CAD build for the part. Positions are in the model's coordinates, mm. Face numbers are marked on the shaded views. A direction names the side the tool comes from. Round coordinates to 2 decimals unless told otherwise and drop trailing zeros. Loops run counter-clockwise (first coordinate to the right, second up) from the corner with the lowest first, then second, coordinate; pieces in that order, holes last.
from build123d import *

# Parameters (mm, degrees)
SKETCH3_W           = 38.1
SKETCH3_H           = 41.932660102
SKETCH3_R           = 7.1501
BOSS_EXTRUDE1_DEPTH = 2.54
SKETCH4_W           = 8.89
SKETCH4_H           = 2.54
BOSS_EXTRUDE2_DEPTH = 8.89


with BuildPart() as part:
    # Sketch3 → Boss-Extrude1 (new body)
    with BuildSketch(Plane(origin=(-73.0954, 0, 0), x_dir=(0, 0, -1), z_dir=(1, 0, 0))):
        with Locations((0, -1.916330051)):
            Rectangle(SKETCH3_W, SKETCH3_H)
        Circle(SKETCH3_R, mode=Mode.SUBTRACT)
    extrude(amount=-BOSS_EXTRUDE1_DEPTH)

    # Sketch4 → Boss-Extrude2 (add)
    with BuildSketch(Plane(origin=(-73.0954, 0, 0), x_dir=(0, 0, -1), z_dir=(1, 0, 0))):
        with Locations((14.605, -21.612660102)):
            Rectangle(SKETCH4_W, SKETCH4_H)
        with Locations((-14.605, -21.612660102)):
            Rectangle(SKETCH4_W, SKETCH4_H)
    extrude(amount=-BOSS_EXTRUDE2_DEPTH)


solid = part.part
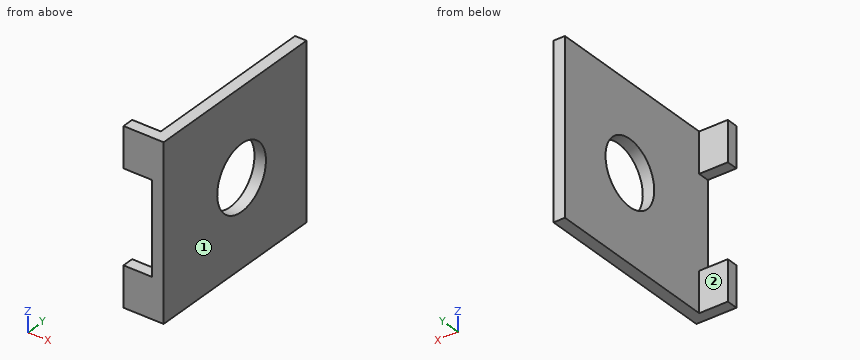
Item 1: Cut at D-D (y = 15.5). List the corners of the cut face in (x, z), plus the area to 3 significant figures.
Verdict:
outline: (-75.64, -19.05) - (-73.1, -19.05) - (-73.1, 19.05) - (-75.64, 19.05) - close
area: 96.8 mm2
Item 2: Wall check: L1, parallel to Y at x = -73.65, z = 0; L2, parallel to X at y = -4, z = 11; L3, parallel to Y at x = -75, z = -6. Give the ranges that are in metal, low to high.
Verdict:
L1: y = -22.88 to -7.15, 7.15 to 19.05
L2: x = -75.64 to -73.1
L3: y = -22.88 to -3.89, 3.89 to 19.05
Item 3: Flat gauge pins, fed straight in: P1, Ø1.9, axis at x = -80, z = -12.5, coming from the +Y side; P2, Ø1, axis at x = -76.5, z = 2.5, coming from the +Y side; P3, Ø1, axis at y = -14.5, z = 10.5, coming from the -X side. Where does each tip first touch, or does it go through?
Verdict:
P1: stops at y = -20.34
P2: passes through
P3: stops at x = -75.64
Item 4: Cut at B-B (z = 0). List the corners of the cut face in (x, y).
Verdict:
outline: (-75.64, -22.88) - (-73.1, -22.88) - (-73.1, -7.15) - (-75.64, -7.15) - close; (-75.64, 7.15) - (-73.1, 7.15) - (-73.1, 19.05) - (-75.64, 19.05) - close
Item 5: Cut at A-A (y = 0). List the corners of the cut face in (x, z), plus the area to 3 significant figures.
Verdict:
outline: (-75.64, -19.05) - (-73.1, -19.05) - (-73.1, -7.15) - (-75.64, -7.15) - close; (-75.64, 7.15) - (-73.1, 7.15) - (-73.1, 19.05) - (-75.64, 19.05) - close
area: 60.5 mm2
Item 6: 3-axis set-ups, long thin cutter, end or side, ignore diameter. For the marked faces 1 and 2: which of +Z, -Z, +X, -X, +Y, -Y reach the whole face in a straight line?
Verdict:
face 1: +Z, -Z, +X, +Y, -Y
face 2: +Z, -Z, -X, +Y
Item 7: Cut at C-C (z = 11). List the corners of the cut face in (x, y), plus the area to 3 significant figures.
Verdict:
outline: (-81.99, -22.88) - (-73.1, -22.88) - (-73.1, 19.05) - (-75.64, 19.05) - (-75.64, -20.34) - (-81.99, -20.34) - close
area: 123 mm2
